CAD build for the part. Positions are in the model's coordinates, mm. Round coordinates to 2 decimals unless told otherwise and drop trailing zeros. Write each loop counter-clockwise with the first axis right and the second up, starting at its lowest first coordinate (ties: lowest second). Pieces come first, ordered by that corner, then holes. Notation, with made-up numbers: (-32, 52.5) -> (-18, 52.5) arc R9 ccw to (-18, 64.5) -> close; hole circle Ø5 at (84.25, 74.25). An arc over 180 degrees is marked (long way). Put each result on its own line as item: value. Start each with the question number.
1. Drill centre lines: line 1 (Z direction, x = -35.5, y = 5); line 2 (Y direction, x = 57, z = 418.5); line 3 (Z direction, x = 6, y = -2.75). Where is each one in solid material? Low to high. Write a range as from..to.
2. Saw through at A-A on y = -5. List the corners of the cut face in (x, z).
3. Saw through at B-B on x = 23. List the corners of the cut face in (y, z), and give its area (3 significant figures).
4. Saw through at D-D on x = 69.5. List the corners of the cut face in (y, z), and give its area (3 significant figures).
5. Flat gauge pins, fed straight in: P1, Ø17, axis at x = 45, z = 443.5, coming from the +Y side; P2, Ø1.5, axis at x = -2, z = 205.5, coming from the -Y side; P3, Ø11, axis at x = 28, y = -3, coming from the -Z side. Where does each tip first touch, or does it go through?
6. Saw through at C-C on z = 383. List the corners of the cut face in (x, y), and give its area (3 significant figures).
from build123d import *

# Parameters (mm, degrees)
F0_R          = 11.4398919201
F1_DEPTH      = 419.01794
F3_DEPTH      = 10.8458
F3_DEPTH_BACK = 10.84517
F4_T2_ANGLE   = 127.5095974459
F4_T4_ANGLE   = 127.5095974459


# Not quite as in the source:
# - a fillet or chamfer that OpenCascade refuses, or shapes differently, is made with other operations: its cross-section is extruded or revolved along the edge and cut away or added


with BuildPart() as f1:
    # F0 (on Top) → F1 (new body)
    with BuildSketch(Plane.XY):
        Circle(F0_R)
    extrude(amount=F1_DEPTH)

    # F2 (on Front) → F3 (join, two sides)
    with BuildSketch(Plane.XZ) as f3_sk:
        with BuildLine():
            Line((-48.4741501155, 456.7061818215), (-48.4741501155, 418.9741480511))
            Line((-48.4741501155, 418.9741480511), (39.7135697317, 418.9741480511))
            Line((39.7135697317, 418.9741480511), (74.8131631411, 413.270452539))
            Line((74.8131631411, 413.270452539), (95.608628696, 403.7768645791))
            ThreePointArc((95.608628696, 403.7768645791), (105.8473453497, 437.8401649363), (95.608628696, 471.9034652936))
            Line((95.608628696, 471.9034652936), (74.8131631411, 462.4098773337))
            Line((74.8131631411, 462.4098773337), (39.7135697317, 456.7061818215))
            Line((39.7135697317, 456.7061818215), (-48.4741501155, 456.7061818215))
        make_face()
    extrude(amount=F3_DEPTH)
    extrude(f3_sk.sketch, amount=-F3_DEPTH_BACK)

    # F4: chamfer of 12.7 on 2 edges, made by hand

    # F4_s1 → F4_t2 (revolve, cut)
    with BuildSketch(Plane(origin=(209.1067778356, 0, 103.0982793805), x_dir=(0, 1, 0), z_dir=(-0.8969097816, 0, -0.4422135724))):
        Polygon((-10.8458, -324.1347521568), (1.8542, -311.4347521568), (-10.8458, -311.4347521568), align=None)
    revolve(axis=Axis((44.0652005391, -10.8458, 437.8401649363), (0, -1, 0)), revolution_arc=F4_T2_ANGLE, mode=Mode.SUBTRACT)

    # F4_s3 → F4_t4 (revolve, cut)
    with BuildSketch(Plane(origin=(209.1067778356, 0, 103.0982793805), x_dir=(0, 1, 0), z_dir=(-0.8969097816, 0, -0.4422135724))):
        Polygon((10.84517, -324.1347521568), (-1.85483, -311.4347521568), (10.84517, -311.4347521568), align=None)
    revolve(axis=Axis((44.0652005391, 10.84517, 437.8401649363), (0, -1, 0)), revolution_arc=F4_T4_ANGLE, mode=Mode.SUBTRACT)


solid = f1.part
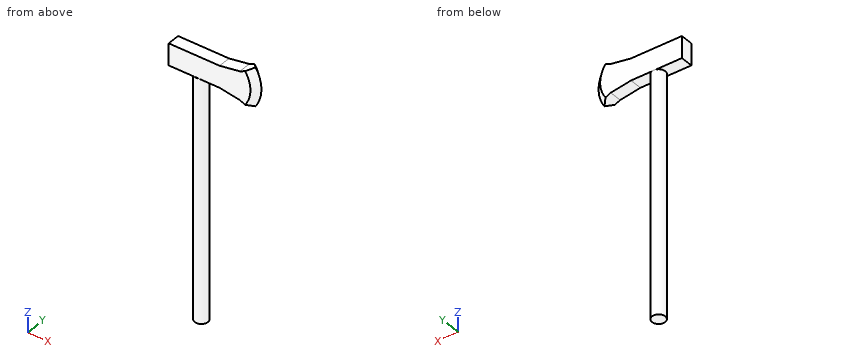
Return value:
1. line 1: z = 418.97..456.71
1. line 2: y = -10.85..10.85
1. line 3: z = 0..456.71
2. outline: (-48.47, 418.97) -> (-10.29, 418.97) -> (-10.29, 0) -> (10.29, 0) -> (10.29, 418.97) -> (39.71, 418.97) -> (74.81, 413.27) -> (89.29, 406.66) arc R54.93 ccw to (89.29, 469.02) -> (74.81, 462.41) -> (39.71, 456.71) -> (-48.47, 456.71) -> close
3. outline: (-10.85, 418.97) -> (10.85, 418.97) -> (10.85, 456.71) -> (-10.85, 456.71) -> close
3. area: 818 mm^2
4. outline: (-10.85, 414.13) -> (10.85, 414.13) -> (10.85, 461.55) -> (-10.85, 461.55) -> close
4. area: 1,030 mm^2
5. P1: stops at y = 10.85
5. P2: stops at y = -11.37
5. P3: stops at z = 418.97
6. outline: circle Ø22.88 at (0, 0)
6. area: 411 mm^2
